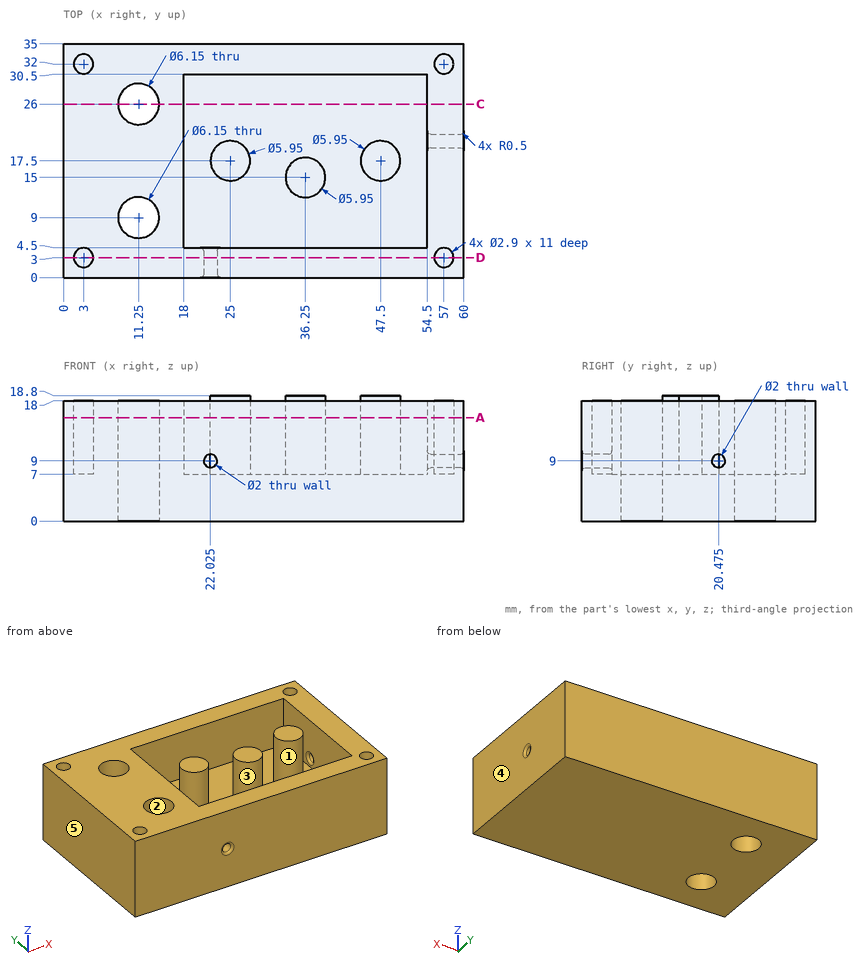
Geometry check sheet. Reference: drawing and pictorial views, mm from the part's lowest x, y, z. A direction names the side the tool comes from. Coordinates: 2 decimals unless noted, no trailing zeros. Loops run counter-clockwise (first coordinate to the right, second up) from the corner with the lowest first, then second, coordinate; pieces in that order, holes last.
1) Sectioned sample at A-A (z = 15.5). Count the separate pieces of the cut face and the enclosed holes in it, and give its area (3 significant figures).
2) Material ranges on probe 1 along Y at (x, z) = (11.25, 13.5) (3 decimals); probe 2 along Y at (x, z) = (36, 17.5); probe 3 along X at (y, z) = (15, 17.25) (3 decimals), recorded low to high.
3) Sectioned sample at C-C (y = 26). Record the boundary of the cut face in (x, z) (3 decimals).
4) Sectioned sample at D-D (y = 3). Record the boundary of the cut face in (x, z) (3 decimals).
5) Gauge pin test, flat ends, axial feed: pin 1 (0.9 mm diameter, centred on x = 57, y = 32.5, fed in from +Z); pin 2 (10 mm diameter, centred on x = 11.25, y = 26, fed in from +Z); pin 3 (1.2 mm diameter, centred on x = 22.025, z = 9, fed in from -Y). Record the tip position at first contact, or that the pin passes through.
6) Access from +Z, -Z, +X, -X, +Y, -Y to the whole of each face (thin tool, end or side, straight path). Record for the marked faces 1 and 2.
7) Release check for a two-part mould opening along X. For the marked faces 3, 4 and 5 record: released by +X, released by -X, zero draft, split by the parting line, or undercut.
Check sheet entries:
1. separate pieces: 4
1. enclosed holes: 7
1. area: 1,150 mm2
2. probe 1: y = 0 to 5.925, 12.075 to 22.925, 29.075 to 35
2. probe 2: y = 0 to 4.5, 12.04 to 17.96, 30.5 to 35
2. probe 3: x = 0 to 18, 23.387 to 26.613, 33.275 to 39.225, 45.887 to 49.113, 54.5 to 60
3. outline: (0, 0) - (8.175, 0) - (8.175, 18) - (0, 18) - close; (14.325, 0) - (60, 0) - (60, 18) - (54.5, 18) - (54.5, 7) - (18, 7) - (18, 18) - (14.325, 18) - close
4. outline: (0, 0) - (60, 0) - (60, 18) - (58.45, 18) - (58.45, 7) - (55.55, 7) - (55.55, 18) - (4.45, 18) - (4.45, 7) - (1.55, 7) - (1.55, 18) - (0, 18) - close; hole circle Ø2 at (22.025, 9)
5. pin 1: stops at z = 7
5. pin 2: stops at z = 18
5. pin 3: stops at y = 15.71
6. face 1: +Z
6. face 2: +Z, -Z
7. face 3: undercut
7. face 4: released by +X
7. face 5: released by -X
